Can you work these out from the model? Positions are in its coordinate system, mm. Face numbers are marked on the shaded views. A direction names the side the tool comes from. Round coordinates to 2 decimals unless told otherwise and drop trailing zeros. Loops run counter-clockwise (first coordinate to the right, second up) from the corner with the lowest first, then second, coordinate; pieces in that order, holes last.
(1) If I drill on line 1 along Y through (x, z) = (0, 0.85); line 2 along Y through (x, z) = (0, 6.25); line 3 along Y through (x, z) = (0, 0.7), over which ranges is the centre line in solid material (lowest first)?
(2) I want a section at B-B on z = 12.5. Write out the boundary of the cut face in (x, y), plus the area to 3 significant figures.
(3) Will these pins go through, and if not, where does the flat tip stop? pin 1 Ø7 at (x, y) = (4, -3.5) entering from +Z; pin 2 Ø5.5 at (x, z) = (14, 9) entering from -Y; pin 3 Ø1 at (x, z) = (-14, 8.5) entering from +Y; pin 4 Ø5 at (x, z) = (6.5, 7) entering from +Y.
(4) I want a section at C-C on z = 7.5. Give the number of separate pieces and of enclosed holes in the cut face, plus the area to 3 significant figures.
(5) Thinking about a two-plate mould opening in Z: for the marked faces 1, 2, 3 and 4, which applies, released by +Z, released by -Z, zero draft, split by the parting line, or undercut?
(6) I want a section at D-D on z = 16.5. Write out the boundary of the cut face in (x, y), plus the area to 3 significant figures.
(7) I want a section at A-A on x = 0. Write out the boundary of the cut face in (y, z).
(8) Which directions (+Z, -Z, +X, -X, +Y, -Y) give clear straight access to the entire face, cutting with the end or side of a thin tool? Please do the marked faces 5, 6, 7, 8 and 9.
from build123d import *

# Parameters (mm, degrees)
SKETCH_R             = 1.2
PAD_DEPTH            = 18
POCKET001_DEPTH      = 0.001
POCKET001_DEPTH_BACK = 18.001
SKETCH001_R          = 11.3
POCKET_DEPTH         = 16.5
SKETCH003_R          = 2.4
POCKET002_DEPTH      = 13
SKETCH004_R          = 2.4
POCKET003_DEPTH      = 13
SKETCH005_W          = 4.2
SKETCH005_H          = 8.4
POCKET004_DEPTH      = 12
SKETCH007_W          = 4.2
SKETCH007_H          = 8.4
POCKET005_DEPTH      = 12
CHAMFER_SIZE         = 1


with BuildPart() as part:
    # Sketch → Pad (new body)
    with BuildSketch(Plane.XY):
        with BuildLine():
            Line((-8.2819133905, -13), (-20.2343664663, 12.6321183381))
            Line((-20.2343664663, 12.6321183381), (-8.4523652348, 18.1261557407))
            ThreePointArc((20, 0), (10.7459921669, 16.8678289163), (-8.4523652348, 18.1261557407))
            Line((20, -13), (20, 0))
            Line((-8.2819133905, -13), (20, -13))
        make_face()
        with Locations((0, 9)):
            Circle(SKETCH_R, mode=Mode.SUBTRACT)
        with Locations((0, -9)):
            Circle(SKETCH_R, mode=Mode.SUBTRACT)
        with Locations((9, 0)):
            Circle(SKETCH_R, mode=Mode.SUBTRACT)
        with Locations((-9, 0)):
            Circle(SKETCH_R, mode=Mode.SUBTRACT)
    extrude(amount=PAD_DEPTH)

    # Sketch002 → Pocket001 (cut, two sides)
    with BuildSketch(Plane.XY) as pocket001_sk:
        with BuildLine():
            Line((-1.7956262222, -6.9724978645), (-6.9724978645, -1.7956262222))
            ThreePointArc((1.7956262222, 6.9724978645), (-5.0911688245, 5.0911688245), (-6.9724978645, -1.7956262222))
            Line((1.7956262222, 6.9724978645), (6.9724978645, 1.7956262222))
            ThreePointArc((-1.7956262222, -6.9724978645), (5.0911688245, -5.0911688245), (6.9724978645, 1.7956262222))
        make_face()
    extrude(amount=-POCKET001_DEPTH, mode=Mode.SUBTRACT)
    extrude(pocket001_sk.sketch, amount=POCKET001_DEPTH_BACK, mode=Mode.SUBTRACT)

    # Sketch001 (on Face11 of Pad) → Pocket (cut)
    with BuildSketch(Plane.XY.offset(18)):
        Circle(SKETCH001_R)
    extrude(amount=-POCKET_DEPTH, mode=Mode.SUBTRACT)

    # Sketch003 (on Face1 of Pocket) → Pocket002 (cut)
    with BuildSketch(Plane(origin=(-11.7820012315, -5.4940374026, 0), x_dir=(0.4226182617, -0.906307787, 0), z_dir=(-0.906307787, -0.4226182617, 0))):
        with Locations((-14, 9)):
            Circle(SKETCH003_R)
    extrude(amount=-POCKET002_DEPTH, mode=Mode.SUBTRACT)

    # Sketch004 (on Face2 of Pocket002) → Pocket003 (cut)
    with BuildSketch(Plane.XZ.offset(13)):
        with Locations((14, 9)):
            Circle(SKETCH004_R)
    extrude(amount=-POCKET003_DEPTH, mode=Mode.SUBTRACT)

    # Sketch005 (on Face5 of Pocket003) → Pocket004 (cut)
    with BuildSketch(Plane(origin=(-8.4523652348, 18.1261557407, 0), x_dir=(-0.906307787, -0.4226182617, 0), z_dir=(-0.4226182617, 0.906307787, 0))):
        with Locations((6.9, 9)):
            Rectangle(SKETCH005_W, SKETCH005_H)
    extrude(amount=-POCKET004_DEPTH, mode=Mode.SUBTRACT)

    # Sketch007 (on Face7 of Pocket004) → Pocket005 (cut)
    with BuildSketch(Plane.YZ.offset(20)):
        with Locations((-6.9, 9)):
            Rectangle(SKETCH007_W, SKETCH007_H)
    extrude(amount=-POCKET005_DEPTH, mode=Mode.SUBTRACT)

    # Chamfer
    chamfer_edges = [part.edges().sort_by_distance(p)[0] for p in [
        (20, -6.5, 0),
        (10.745992, 16.867829, 0),
        (5.859043, -13, 0),
        (-14.25814, -0.183941, 0),
        (-14.343366, 15.379137, 0),
    ]]
    chamfer(chamfer_edges, length=CHAMFER_SIZE)


solid = part.part
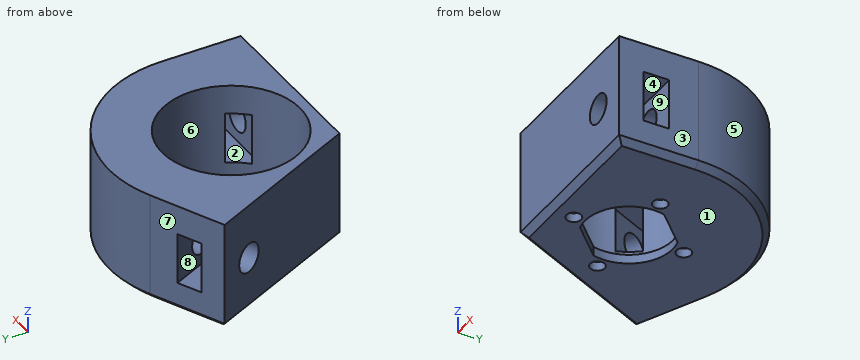
Filled sheet:
1. line 1: y = -12.85 to -10.2, -7.8 to -7.2, 7.2 to 7.8, 10.2 to 19.85
1. line 2: y = -13 to -11.3, 11.3 to 20
1. line 3: y = -12.7 to -10.2, -7.8 to -7.2, 7.2 to 7.8, 10.2 to 19.7
2. outline: (-20.23, 12.63) - (-8.28, -13) - (20, -13) - (20, -9) - (8, -9) - (8, -7.98) arc R11.3 cw to (-10.61, 3.88) - (-11.54, 3.45) - (-16.61, 14.32) - close; (-12.8, 16.1) - (-8.67, 7.24) arc R11.3 cw to (10.23, -4.8) - (20, -4.8) - (20, 0) arc R20 ccw to (-8.45, 18.13) - close
2. area: 535 mm2
3. pin 1: stops at z = 1.5
3. pin 2: stops at y = -13
3. pin 3: stops at y = 6.61
3. pin 4: stops at y = 19.6
4. separate pieces: 4
4. enclosed holes: 0
4. area: 469 mm2
5. face 1: released by -Z
5. face 2: undercut
5. face 3: zero draft
5. face 4: undercut
6. outline: (-20.23, 12.63) - (-8.28, -13) - (20, -13) - (20, 0) arc R20 ccw to (-8.45, 18.13) - close; hole circle Ø22.6 at (0, 0)
6. area: 628 mm2
7. outline: (-13, 1) - (-12, 0) - (-10.2, 0) - (-10.2, 1.5) - (-11.3, 1.5) - (-11.3, 18) - (-13, 18) - close; (-7.8, 0) - (-7.2, 0) - (-7.2, 1.5) - (-7.8, 1.5) - close; (7.2, 0) - (7.8, 0) - (7.8, 1.5) - (7.2, 1.5) - close; (10.2, 0) - (19, 0) - (20, 1) - (20, 18) - (11.3, 18) - (11.3, 1.5) - (10.2, 1.5) - close
8. face 5: +Z, -Z, +Y
8. face 6: +Z
8. face 7: +Z, -Z, -X, +Y
8. face 8: none
8. face 9: +X
